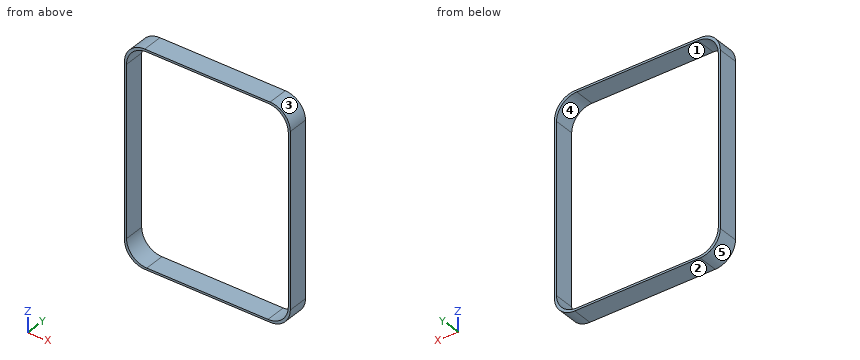
from build123d import *

# Parameters (mm, degrees)
BOX028_W     = 80
BOX028_H     = 10
BOX028_DEPTH = 103.5
FILLET033_R  = 10
BOX029_W     = 82
BOX029_H     = 10
BOX029_DEPTH = 105.5
FILLET034_R  = 10


with BuildPart() as obj1:
    # Box028 → Box028 (new body)
    with BuildSketch(Plane(origin=(-1, -26, -14.75), x_dir=(1, 0, 0), z_dir=(0, 0, 1))):
        with Locations((40, 5)):
            Rectangle(BOX028_W, BOX028_H)
    extrude(amount=BOX028_DEPTH)

    # Fillet033
    fillet033_edges = [obj1.edges().sort_by_distance(p)[0] for p in [
        (-1, -21, 88.75),
        (-1, -21, -14.75),
        (79, -21, 88.75),
        (79, -21, -14.75),
    ]]
    fillet(fillet033_edges, radius=FILLET033_R)


with BuildPart() as obj1_1:
    # Fillet033 placement: moved
    add(obj1.part.moved(Location((0, 0.5, 0))))


with BuildPart() as topcut:
    # Box029 → Box029 (new body)
    with BuildSketch(Plane(origin=(-2, -27, -15.75), x_dir=(1, 0, 0), z_dir=(0, 0, 1))):
        with Locations((41, 5)):
            Rectangle(BOX029_W, BOX029_H)
    extrude(amount=BOX029_DEPTH)

    # Fillet034
    fillet034_edges = [topcut.edges().sort_by_distance(p)[0] for p in [
        (-2, -22, 89.75),
        (-2, -22, -15.75),
        (80, -22, 89.75),
        (80, -22, -15.75),
    ]]
    fillet(fillet034_edges, radius=FILLET034_R)


with BuildPart() as topcut_1:
    # Fillet034 placement: moved
    add(topcut.part.moved(Location((0, 1.5, 0))))

    # Cut009: cut obj1
    add(obj1_1.part, mode=Mode.SUBTRACT)


solid = topcut_1.part
Design review of the part built by this model. Coordinates are the model's own, in mm. Face numbers are marked on the shaded views. A direction names the side the tool comes from. Round coordinates to 2 decimals unless told otherwise and drop trailing zeros. Order: outer loops, then holes, each group sorted by start corner. A loop starts at its lowest first (then second) coordinate and runs counter-clockwise, first axis right, second up.
1) Consider section B-B (x = 40.5). State the section outline as (y, z) points.
The answers:
outline: (-25.5, -15.75) - (-15.5, -15.75) - (-15.5, -14.75) - (-25.5, -14.75) - close; (-25.5, 88.75) - (-15.5, 88.75) - (-15.5, 89.75) - (-25.5, 89.75) - close
2) Draft analysis for pull direction X (two halves, no side actions). For the marked faces 3, 4 and 5, state which applies: released by +X, released by -X, zero draft, split by the parting line, or undercut.
The answers:
face 3: released by +X
face 4: undercut
face 5: released by -X
3) For L1, parallel to Z at x = 55.5, y = -21.5; L2, parallel to X at y = -16.75, z = 71; L3, parallel to Z at x = 8, y = -22, list the stretches that pass through material, from the lowest coordinate up.
The answers:
L1: z = -15.75 to -14.75, 88.75 to 89.75
L2: x = -2 to -1, 79 to 80
L3: z = -15.75 to -14.7, 88.7 to 89.75
4) Consider section A-A (y = -17). State the section outline as (x, z) points, plus the area to 3 significant figures.
The answers:
outline: (-2, -5.75) arc R10 ccw to (8, -15.75) - (70, -15.75) arc R10 ccw to (80, -5.75) - (80, 79.75) arc R10 ccw to (70, 89.75) - (8, 89.75) arc R10 ccw to (-2, 79.75) - close; hole (-1, -4.75) arc R10 ccw to (9, -14.75) - (69, -14.75) arc R10 ccw to (79, -4.75) - (79, 78.75) arc R10 ccw to (69, 88.75) - (9, 88.75) arc R10 ccw to (-1, 78.75) - close
area: 371 mm2
5) Consider section C-C (z = 29). State the section outline as (x, y) points, plus the area to 3 significant figures.
The answers:
outline: (-2, -25.5) - (-1, -25.5) - (-1, -15.5) - (-2, -15.5) - close; (79, -25.5) - (80, -25.5) - (80, -15.5) - (79, -15.5) - close
area: 20.0 mm2
6) Machinability: for the marked faces 1 and 2, which of the approach directions +Z, -Z, +X, -X, +Y, -Y give a long, thin tool a straight path to every point of the face, cutting with its end or side? Answer none if there is none.
The answers:
face 1: +Y, -Y
face 2: -Z, +X, -X, +Y, -Y
